from build123d import *

# Parameters (mm, degrees)
F0_R     = 6
F1_DEPTH = 60
F2_R     = 7
F3_R     = 3.1
F4_DEPTH = 8.001


with BuildPart() as f1:
    # F0 (on Front) → F1 (new body)
    with BuildSketch(Plane.XZ):
        with BuildLine():
            Line((-30, -8), (-7.141428, -8))
            ThreePointArc((-7.141428, -8), (0, -25), (7.141428, -8))
            Line((7.141428, -8), (30, -8))
            Line((30, -8), (30, 0))
            Line((30, 0), (-30, 0))
            Line((-30, 0), (-30, -8))
        make_face()
        with Locations((0, -15)):
            Circle(F0_R, mode=Mode.SUBTRACT)
    extrude(amount=-F1_DEPTH)

    # F2
    f2_edges = [f1.edges().sort_by_distance(p)[0] for p in [
        (7.141428, 30, -8),
        (-7.141428, 30, -8),
    ]]
    fillet(f2_edges, radius=F2_R)

    # F3 (on face) → F4 (cut, through all)
    with BuildSketch(Plane(origin=(0, 0, -8), x_dir=(1, 0, 0), z_dir=(0, 0, -1))):
        with Locations((-23, -7)):
            Circle(F3_R)
        with Locations((-23, -53)):
            Circle(F3_R)
        with Locations((23, -7)):
            Circle(F3_R)
        with Locations((23, -53)):
            Circle(F3_R)
    extrude(amount=-F4_DEPTH, mode=Mode.SUBTRACT)


solid = f1.part
Source: CAD feature listing. Evaluate the final solid. Frame: model axes, mm. A direction names the side the tool comes from. Give positions to 0.01 mm unless a question says otherwise; leave off trailing zeros. Write each loop counter-clockwise with the first axis right and the second up, starting at its lowest first coordinate (ties: lowest second). Pieces come first, ordered by that corner, then holes. Notation, with made-up numbers: M 7,-17 L 23,-17 A21 ccw 23,18 Z; hole C 41.5,57 d11. An arc over 180 degrees is marked long. Return JSON: item names as keys, results as strings. Group by question number.
1) Pull-direction query (Y, two-part tool) for faces 1 (the face through (19.9, 6.9, -4.1)), 2 (the face through (12, 30.4, -10.1)), 3 (the face through (0, 60, -7)); classes: pulls with the +Y half, pulls with the -Y half, needs draft (parallel to the pull), parting line crosses it, or undercut.
2) Pin query (flat end, axial travel): P1, Ø1, axis at y = 45.5, z = -20, coming from the +X side; P2, Ø6.5, axis at x = 25, y = 21.5, coming from the -Z side. Return the tip coordinate at first contact, or that it passes through.
3) Cut plane B-B, the plane y = 7. Output: boundary loops of the cut face in (x, z), plus the area to 3 significant figures.
4) Cut plane A-A, the plane x = 23. Output: boundary loops of the cut face in (y, z), plus the area to 3 significant figures.
5) Cut plane D-D, the plane z = -4.75. Output: boundary loops of the cut face in (x, y).
6) Cut plane C-C, the plane x = 0. Output: boundary loops of the cut face in (y, z).
7) Set-up query: faces 4 (the face through (-24, 30, -8)), 5 (the face through (-23.404, 49.926, -4.056)), 6 (the face through (23, 30, -8)). Return all of +Z, -Z, +X, -X, +Y, -Y with unobstructed straight access to the full face (end or side cutting, diameter ignored); none if empty.
8) Material intervals for line 1 along X through (y, z) = (53, -2.5); line 2 along Y through (x, z) = (23, -2.5); line 3 along Z through (x, y) = (0, 34), sorted ascending. Write a range as [from, to].
Recorded:
{
 "1": {"face 1": "undercut", "face 2": "needs draft", "face 3": "pulls with the +Y half"},
 "2": {"P1": "stops at x = 8.93", "P2": "stops at z = -8"},
 "3": {"outline": "M -30,-8 L -26.1,-8 L -26.1,0 L -30,0 Z; M -19.9,-8 L -17,-8 A7 cw -10,-15 A10 ccw 10,-15 A7 cw 17,-8 L 19.9,-8 L 19.9,0 L -19.9,0 Z; M 26.1,-8 L 30,-8 L 30,0 L 26.1,0 Z; hole C 0,-15 d12", "area": "586 mm²"},
 "4": {"outline": "M 0,-8 L 3.9,-8 L 3.9,0 L 0,0 Z; M 10.1,-8 L 49.9,-8 L 49.9,0 L 10.1,0 Z; M 56.1,-8 L 60,-8 L 60,0 L 56.1,0 Z", "area": "381 mm²"},
 "5": {"outline": "M -30,0 L 30,0 L 30,60 L -30,60 Z; hole C -23,7 d6.2; hole C -23,53 d6.2; hole C 23,7 d6.2; hole C 23,53 d6.2"},
 "6": {"outline": "M 0,-25 L 60,-25 L 60,-21 L 0,-21 Z; M 0,-9 L 60,-9 L 60,0 L 0,0 Z"},
 "7": {"face 4": "-Z, -X, +Y, -Y", "face 5": "+Z, -Z", "face 6": "-Z, +X, +Y, -Y"},
 "8": {"line 1": "x = [-30, -26.1], [-19.9, 19.9], [26.1, 30]", "line 2": "y = [0, 3.9], [10.1, 49.9], [56.1, 60]", "line 3": "z = [-25, -21], [-9, 0]"}
}
